Check sheet for the drawn part. Datum: minimum x, y, z corner. Units: mm. A direction names the side the tool comes from. Round coordinates to 2 decimals unless told otherwise and drop trailing zeros. Loops run counter-clockwise (first coordinate to the right, second up) from the corner with the lowest first, then second, coordinate; pieces in that order, holes last.
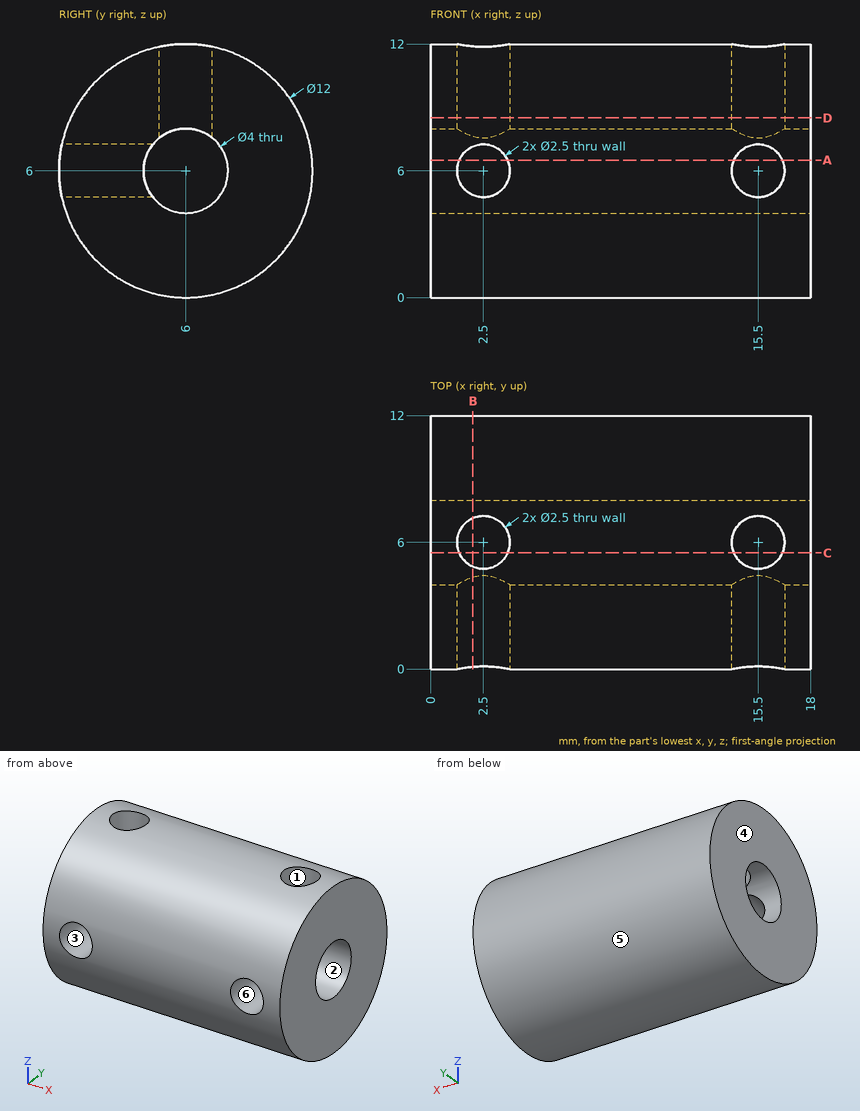
1) Sectioned sample at D-D, the plane z = 8.5. Record the cut outline in (x, y), then the cut area to 3 significant figures.
Report:
outline: (0, 0.55) - (18, 0.55) - (18, 11.45) - (0, 11.45) - close; hole circle Ø2.5 at (2.5, 6); hole circle Ø2.5 at (15.5, 6)
area: 187 mm2
2) Scan lines: line 1 along Y through (x, z) = (13.5, 6); line 2 along X through (y, z) = (5.75, 10.5); line 3 along Z through (x, y) = (1, 5.5). Record each from-to range of solid material in increasing order.
Report:
line 1: y = 0 to 4, 8 to 12
line 2: x = 0 to 1.28, 3.72 to 14.28, 16.72 to 18
line 3: z = 0.02 to 4.06, 7.94 to 11.98
3) Sectioned sample at C-C, the plane y = 5.5. Record the cut outline in (x, z), then the cut area to 3 significant figures.
Report:
outline: (0, 0.02) - (18, 0.02) - (18, 4.06) - (0, 4.06) - close; (0, 7.94) - (1.35, 7.94) - (1.35, 11.98) - (0, 11.98) - close; (3.65, 7.94) - (14.35, 7.94) - (14.35, 11.98) - (3.65, 11.98) - close; (16.65, 7.94) - (18, 7.94) - (18, 11.98) - (16.65, 11.98) - close
area: 127 mm2
4) Gauge pin test, flat end, axial feed: pin 1 (1.5 mm diameter, centred on x = 7.5, z = 4, fed in from -Y). Record the tip position at first contact, or that the pin passes through.
Report:
pin 1: stops at y = 0.13
5) Access from +Z, -Z, +X, -X, +Y, -Y to the whole of each face (thin tool, end or side, straight path). Record for the marked faces 1, 2 and 3.
Report:
face 1: +Z
face 2: +X, -X
face 3: -Y
6) Mould release check, pull along Z, two halves, no side actions. Record for the marked faces 4, 5 and 6: +Z half, -Z half, draft (parallel to the pull), parting line (faces both ways), or undercut.
Report:
face 4: draft
face 5: parting line
face 6: undercut
7) Sectioned sample at B-B, the plane x = 2. Record the cut outline in (y, z), then the cut area to 3 significant figures.
Report:
outline: (0.11, 4.85) arc R6 ccw (long way) to (7.15, 11.89) - (7.15, 7.64) arc R2 cw (long way) to (4.36, 4.85) - close; (0.11, 7.15) - (4.36, 7.15) arc R2 cw to (4.85, 7.64) - (4.85, 11.89) arc R6 ccw to start
area: 81.8 mm2
8) Sectioned sample at A-A, the plane z = 6.5. Record the cut outline in (x, y).
Report:
outline: (0, 0.02) - (1.35, 0.02) - (1.35, 4.06) - (0, 4.06) - close; (0, 7.94) - (18, 7.94) - (18, 11.98) - (0, 11.98) - close; (3.65, 0.02) - (14.35, 0.02) - (14.35, 4.06) - (3.65, 4.06) - close; (16.65, 0.02) - (18, 0.02) - (18, 4.06) - (16.65, 4.06) - close
